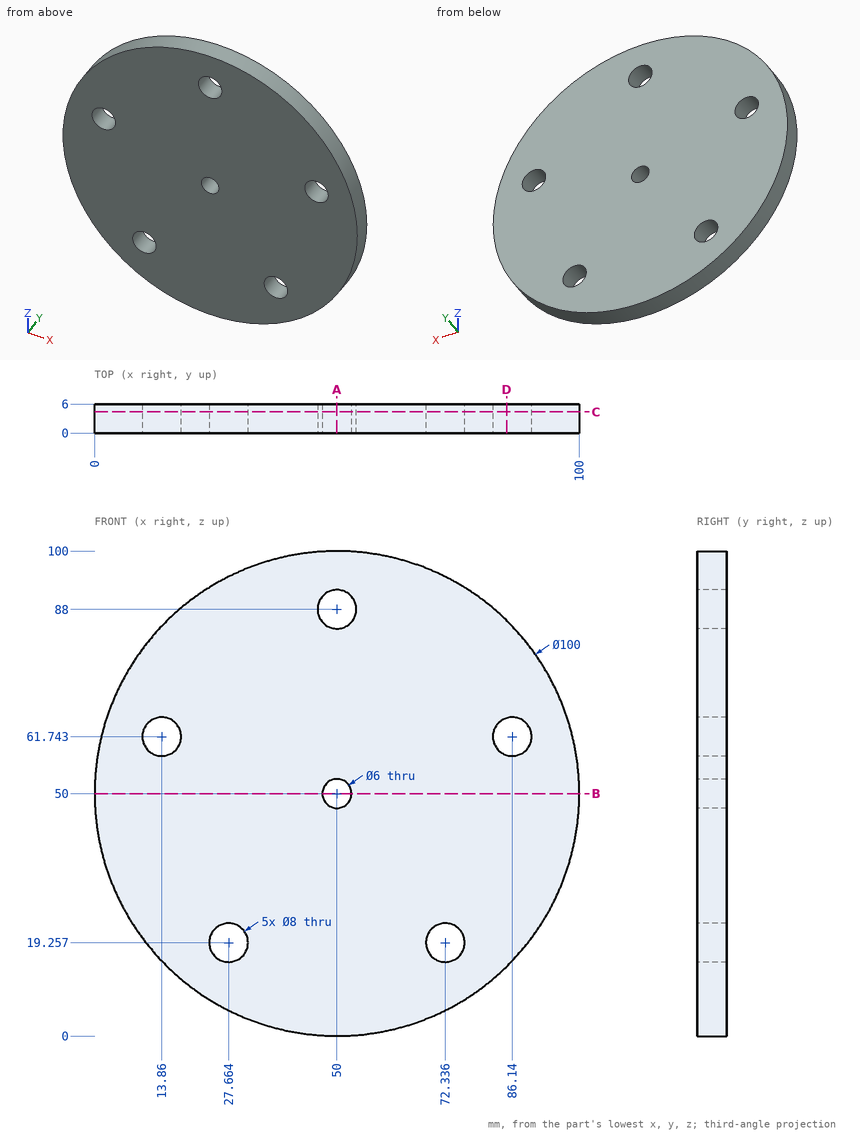
Here's the drawing with two shaded views (mm, measured from the low corner). I have some questions. Give positions to 0.01 mm unless a question says otherwise; leave off trailing zeros. Order: outer loops, then holes, each group sorted by start corner. A loop starts at its lowest first (then second) coordinate and runs counter-clockwise, first axis right, second up. Notation, with made-up numbers: (-4.5, 58) - (2.5, 58) arc R28 cw to (2.5, 82) - close; hole circle Ø1 at (19, -16). An arc over 180 degrees is marked (long way). Use a Markdown table: item, result. Add a question column.
Q1. If we section it at D-D on x = 85: Write out the boundary of the cut face in (y, z).
Q2. If we section it at B-B on z = 50: Write out the boundary of the cut face in (x, y), plus the area to 3 significant figures.
Q3. If we section it at A-A on x = 50: Write out the boundary of the cut face in (y, z).
Q4. Please list where these lines run through material, in increasing order: line 1 along Z through (x, y) = (50, 2.25); line 2 along X through (y, z) = (1.7, 59.5); line 3 along X through (y, z) = (2.35, 61) (1 decimal).
Q5. If we section it at C-C on y = 4.4: Write out the boundary of the cut face in (x, z).
Q6. I'm going to push flat-ended pins straight in: pin 1 (1.5 mm diameter, centred on x = 54, y = 4.5, fed in from +Z); pin 2 (3 mm diameter, centred on x = 40, y = 5.5, fed in from +Z); pin 3 (1 mm diameter, centred on y = 3, z = 53, fed in from +X). Where does each tip first touch, or does it pass through?
Answers follow:
| question | item | result |
|---|---|---|
| 1 | outline | (0, 14.29) - (6, 14.29) - (6, 57.91) - (0, 57.91) - close; (0, 65.58) - (6, 65.58) - (6, 85.71) - (0, 85.71) - close |
| 2 | outline | (0, 0) - (47, 0) - (47, 6) - (0, 6) - close; (53, 0) - (100, 0) - (100, 6) - (53, 6) - close |
| 2 | area | 564 mm^2 |
| 3 | outline | (0, 0) - (6, 0) - (6, 47) - (0, 47) - close; (0, 53) - (6, 53) - (6, 84) - (0, 84) - close; (0, 92) - (6, 92) - (6, 100) - (0, 100) - close |
| 4 | line 1 | z = 0 to 47, 53 to 84, 92 to 100 |
| 4 | line 2 | x = 0.91 to 10.55, 17.17 to 82.83, 89.45 to 99.09 |
| 4 | line 3 | x = 1.2 to 9.9, 17.8 to 82.2, 90.1 to 98.8 |
| 5 | outline | circle Ø100 at (50, 50); hole circle Ø8 at (13.86, 61.74); hole circle Ø8 at (27.66, 19.26); hole circle Ø8 at (50, 88); hole circle Ø6 at (50, 50); hole circle Ø8 at (72.34, 19.26); hole circle Ø8 at (86.14, 61.74) |
| 6 | pin 1 | stops at z = 99.89 |
| 6 | pin 2 | stops at z = 99.27 |
| 6 | pin 3 | stops at x = 99.94 |
